from build123d import *

# Parameters (mm, degrees)
F0_R      = 7.25
F1_DEPTH  = 3.8
F2_R      = 1.45
F3_DEPTH  = 1.5
F3_TAPER  = 3
F8_DEPTH  = 3
F10_DEPTH = 2.5
F10_TAPER = 3
F11_R     = 0.5
F12_SIZE  = 0.5


# Not quite as in the source:
# - a fillet or chamfer that OpenCascade refuses, or shapes differently, is made with other operations: its cross-section is extruded or revolved along the edge and cut away or added


with BuildPart() as f1:
    # F0 (on Top) → F1 (new body)
    with BuildSketch(Plane.XY):
        Circle(F0_R)
    extrude(amount=F1_DEPTH)

    # F2 (on face) → F3 (join)
    with BuildSketch(Plane.XY.offset(3.8)):
        with Locations((0, 5)):
            Circle(F2_R)
        with Locations((0, -5)):
            Circle(F2_R)
    extrude(amount=F3_DEPTH, taper=F3_TAPER)

    # F4: chamfer of 0.5 on 2 edges, made by hand

    # F4_s1 → F4_t2 (revolve, cut)
    with BuildSketch(Plane.XZ.offset(-5)):
        Polygon((1.3975563092, 4.8006852326), (0.8713883311, 5.3), (1.3713883311, 5.3), align=None)
    revolve(axis=Axis((0, 5, 5.3), (0, 0, -1)), mode=Mode.SUBTRACT)

    # F4_s3 → F4_t4 (revolve, cut)
    with BuildSketch(Plane.XZ.offset(5)):
        Polygon((1.3975563092, 4.8006852326), (0.8713883311, 5.3), (1.3713883311, 5.3), align=None)
    revolve(axis=Axis((0, -5, 5.3), (0, 0, -1)), mode=Mode.SUBTRACT)

    # F5 (on Right) → F6 (revolve, cut)
    with BuildSketch(Plane.YZ):
        with BuildLine():
            add(Edge.make_bspline(
                [(0, 3.2), (-3, 3.2), (-6.75, 2.5), (-6.75, 0)],
                knots=[0, 0, 0, 0, 7.4701070943, 7.4701070943, 7.4701070943, 7.4701070943], degree=3))
            Line((-6.75, 0), (0, 0))
            Line((0, 0), (0, 3.2))
        make_face()
    revolve(axis=Axis((0, 0, 2.9542176053), (0, 0, 1)), mode=Mode.SUBTRACT)

    # F7 (on face) → F8 (join)
    with BuildSketch(Plane.XY):
        with BuildLine():
            Line((-1.5, 6.5812232905), (-1.5, -6.5812232905))
            ThreePointArc((-1.5, -6.5812232905), (0, -6.75), (1.5, -6.5812232905))
            Line((1.5, -6.5812232905), (1.5, 6.5812232905))
            ThreePointArc((1.5, 6.5812232905), (0, 6.75), (-1.5, 6.5812232905))
        make_face()
    extrude(amount=F8_DEPTH)

    # F9 (on face) → F10 (cut)
    with BuildSketch(Plane(origin=(0, 0, 0), x_dir=(1, 0, 0), z_dir=(0, 0, -1))):
        with BuildLine():
            ThreePointArc((0.75, 4.25), (0, 5), (-0.75, 4.25))
            Line((-0.75, 4.25), (-0.75, -4.25))
            ThreePointArc((-0.75, -4.25), (0, -5), (0.75, -4.25))
            Line((0.75, -4.25), (0.75, 4.25))
        make_face()
    extrude(amount=-F10_DEPTH, taper=F10_TAPER, mode=Mode.SUBTRACT)

    # F11
    f11_edges = [f1.edges().sort_by_distance(p)[0] for p in [
        (0, -4.868981, 2.5),
        (-0.618981, 0, 2.5),
        (0, 4.868981, 2.5),
        (0.618981, 0, 2.5),
    ]]
    fillet(f11_edges, radius=F11_R)

    # F12
    f12_edges = [f1.edges().sort_by_distance(p)[0] for p in [
        (-7.25, 0, 3.8),
    ]]
    chamfer(f12_edges, length=F12_SIZE)


solid = f1.part
Design review of the part built by this model. Coordinates are the model's own, in mm. A direction names the side the tool comes from. Round coordinates to 2 decimals unless told otherwise and drop trailing zeros. Write each loop counter-clockwise with the first axis right and the second up, starting at its lowest first coordinate (ties: lowest second). Pieces come first, ordered by that corner, then holes. Notation, with made-up numbers: M -4.5,22 L 51.5,22 A16 ccw 51.5,52 Z; hole C 13.5,69.25 d8. An arc over 180 degrees is marked long. One line per item, written item: value. Start each with the question number.
1. Take a section at B-B on z = 0.6. State how many separate pieces and enclosed holes the cut face has, then the cut area to 3 significant figures.
2. Take a section at A-A on z = 3.55. State the section outline as (x, y) points.
3. Draft analysis for pull direction Y (two halves, no side actions). For faces 1 (the face through (0, -5, 5.3)), 2 (the face through (3.35, -6.43, 1.63)), 3 (the face through (-0.307, -6.384, 4.419)), state which applies: pulls with the +Y half, pulls with the -Y half, needs draft (parallel to the pull), parting line crosses it, or undercut.
4. Clearance check with flat-ended pins moving along their axes: P1, Ø2, axis at x = -1, y = -3, coming from the +Z side; P2, Ø1.5, axis at x = -0.5, y = -0.5, coming from the +Z side; P3, Ø0.9, axis at y = 2, z = 1, coming from the +X side. State where each tip first meets the part, or that it passes through.
5. To check wall thickness, follow probe 1 along X at (y, z) = (-1.25, 0.65); probe 2 along X at (y, z) = (2.25, 1.55); probe 3 along X at (y, z) = (5.25, 0.5). State the ranges of each line that lie inside material, in increasing order. Write a range as from..to.
6. For faces 4 (the face through (0, 0, 3.8)), 5 (the face through (0, 5, 5.3)), 6 (the face through (0, 0, 3)), 7 (the face through (0.696, 0.059, 1.027)), list the 3-axis set-ups (+Z, -Z, +X, -X, +Y, -Y) from which the entire face can be reached by the end or side of a thin tool; tool diameter is ignored.
Computed:
1. separate pieces: 1
1. enclosed holes: 3
1. area: 51.2 mm²
2. outline: C 0,0 d14
3. face 1: needs draft
3. face 2: parting line crosses it
3. face 3: undercut
4. P1: stops at z = 4.95
4. P2: stops at z = 3.8
4. P3: stops at x = 7.08
5. probe 1: x = -7.14..-6.54, -1.5..-0.72, 0.72..1.5, 6.54..7.14
5. probe 2: x = -6.89..-5.69, -1.5..-0.67, 0.67..1.5, 5.69..6.89
5. probe 3: x = -5..-4.16, -1.5..1.5, 4.16..5
6. face 4: +Z
6. face 5: +Z, +X, -X, +Y, -Y
6. face 6: none
6. face 7: -Z
